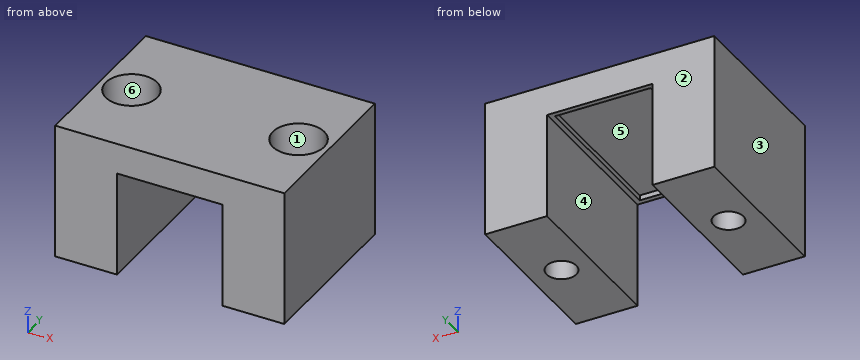
from build123d import *

# Parameters (mm, degrees)
SKETCH1_W                                           = 44.5
SKETCH1_H                                           = 32.2
BOSS_EXTRUDE1_DEPTH                                 = 6
SKETCH2_W                                           = 12
SKETCH2_H                                           = 32.2
BOSS_EXTRUDE2_DEPTH                                 = 20.5
CBORE_FOR_M5_HEX_SOCKET_HEAD_CAP_SCREW1_D           = 5.8
CBORE_FOR_M5_HEX_SOCKET_HEAD_CAP_SCREW1_CBORE_D     = 10
CBORE_FOR_M5_HEX_SOCKET_HEAD_CAP_SCREW1_CBORE_DEPTH = 7.4
SKETCH6_W                                           = 18.5
SKETCH6_H                                           = 30.2
CUT_EXTRUDE1_DEPTH                                  = 1


with BuildPart() as part:
    # Sketch1 → Boss-Extrude1 (new body)
    with BuildSketch(Plane.XY):
        with Locations((22.25, 16.1)):
            Rectangle(SKETCH1_W, SKETCH1_H)
    extrude(amount=BOSS_EXTRUDE1_DEPTH)

    # Sketch2 → Boss-Extrude2 (add)
    with BuildSketch(Plane(origin=(0, 0, 0), x_dir=(-1, 0, 0), z_dir=(0, 0, -1))):
        with Locations((-38.5, 16.1)):
            Rectangle(SKETCH2_W, SKETCH2_H)
        with Locations((-6, 16.1)):
            Rectangle(SKETCH2_W, SKETCH2_H)
    extrude(amount=BOSS_EXTRUDE2_DEPTH)

    # CBORE for M5 Hex Socket Head Cap Screw1 (through all)
    with Locations(Plane.XY.offset(6)):
        with Locations((6.025, 16.1), (38.475, 16.1)):
            CounterBoreHole(CBORE_FOR_M5_HEX_SOCKET_HEAD_CAP_SCREW1_D / 2, CBORE_FOR_M5_HEX_SOCKET_HEAD_CAP_SCREW1_CBORE_D / 2, CBORE_FOR_M5_HEX_SOCKET_HEAD_CAP_SCREW1_CBORE_DEPTH)

    # Sketch6 → Cut-Extrude1 (cut)
    with BuildSketch(Plane(origin=(0, 0, 0), x_dir=(-1, 0, 0), z_dir=(0, 0, -1))):
        with Locations((-22.25, 16.1)):
            Rectangle(SKETCH6_W, SKETCH6_H)
    extrude(amount=-CUT_EXTRUDE1_DEPTH, mode=Mode.SUBTRACT)


solid = part.part
Can you work these out from the model? Positions are in its coordinate system, mm. Face numbers are marked on the shaded views. A direction names the side the tool comes from. Give positions to 0.01 mm unless a question says otherwise; leave off trailing zeros. Write each loop counter-clockwise with the first axis right and the second up, starting at its lowest first coordinate (ties: lowest second). Pieces come first, ordered by that corner, then holes. Notation, with made-up numbers: (23.25, 16.25) -> (50.25, 16.25) arc R29 ccw to (50.25, 40.25) -> close; hole circle Ø11 at (57, 59). An arc over 180 degrees is marked (long way). Answer as a JSON object with one key per item and string values. Group by question number.
Item 1: For the marked faces 4, 5 and 6, which set-ups out of +Z, -Z, +X, -X, +Y, -Y let a thin tool reach every point of the face, with its end or its side?
Item 2: Suppose I cut it at A-A (z = -2.5). Please give me the cut outline in (x, y) (3 decimals), plus the area to 3 significant figures.
Item 3: Please list where these lines run through material, in increasing order: line 1 (X direction, y = 5, z = -4); line 2 (X direction, y = 13.5, z = -12.5); line 3 (Z direction, x = 26, y = 8.5). Write a range as [from, to].
Item 4: We'd pull the mould along X, two halves only. Please class the marked faces 1, 2 and 3: +X half, -X half, draft (parallel to the pull), parting line (faces both ways), or undercut.
Item 5: I'm going to push flat-ended pins straight in: P1, Ø9, axis at x = 19, y = 14, coming from the -Z side; P2, Ø5, axis at x = 6.025, y = 16.1, coming from the +Z side; P3, Ø9, axis at x = 38.475, y = 16.1, coming from the +Z side. Where does each tip first touch, or does it pass through?
Item 6: Suppose I cut it at C-C (x = 38.5). Please give me the cut outline in (y, z), plus the area to 3 significant figures.
Item 7: Suppose I cut it at D-D (y = 23). Please give me the cut outline in (x, z), plus the area to 4 significant figures.
Item 8: Suppose I cut it at B-B (y = 16.1). Please give me the cut outline in (x, z) (3 decimals), plus the area to 3 significant figures.
Findings:
{
 "1": {"face 4": "-Z, +Y, -Y", "face 5": "-Z", "face 6": "+Z"},
 "2": {"outline": "(0, 0) -> (12, 0) -> (12, 32.2) -> (0, 32.2) -> close; (32.5, 0) -> (44.5, 0) -> (44.5, 32.2) -> (32.5, 32.2) -> close; hole circle Ø5.8 at (6.025, 16.1); hole circle Ø5.8 at (38.475, 16.1)", "area": "720 mm²"},
 "3": {"line 1": "x = [0, 12], [32.5, 44.5]", "line 2": "x = [0, 4.74], [7.31, 12], [32.5, 37.19], [39.76, 44.5]", "line 3": "z = [1, 6]"},
 "4": {"face 1": "undercut", "face 2": "draft", "face 3": "-X half"},
 "5": {"P1": "stops at z = 1", "P2": "passes through", "P3": "stops at z = -1.4"},
 "6": {"outline": "(0, -20.5) -> (13.2, -20.5) -> (13.2, -1.4) -> (11.1, -1.4) -> (11.1, 6) -> (0, 6) -> close; (19, -20.5) -> (32.2, -20.5) -> (32.2, 6) -> (21.1, 6) -> (21.1, -1.4) -> (19, -1.4) -> close", "area": "669 mm²"},
 "7": {"outline": "(0, -20.5) -> (12, -20.5) -> (12, 0) -> (13, 0) -> (13, 1) -> (31.5, 1) -> (31.5, 0) -> (32.5, 0) -> (32.5, -20.5) -> (44.5, -20.5) -> (44.5, 6) -> (0, 6) -> close", "area": "740.5 mm²"},
 "8": {"outline": "(0, -20.5) -> (3.125, -20.5) -> (3.125, -1.4) -> (1.025, -1.4) -> (1.025, 6) -> (0, 6) -> close; (8.925, -20.5) -> (12, -20.5) -> (12, 0) -> (13, 0) -> (13, 1) -> (31.5, 1) -> (31.5, 0) -> (32.5, 0) -> (32.5, -20.5) -> (35.575, -20.5) -> (35.575, -1.4) -> (33.475, -1.4) -> (33.475, 6) -> (11.025, 6) -> (11.025, -1.4) -> (8.925, -1.4) -> close; (41.375, -20.5) -> (44.5, -20.5) -> (44.5, 6) -> (43.475, 6) -> (43.475, -1.4) -> (41.375, -1.4) -> close", "area": "371 mm²"}
}
